from build123d import *

# Parameters (mm, degrees)
PAD_DEPTH = 3


with BuildPart() as part:
    # Sketch → Pad (new body, symmetric)
    with BuildSketch(Plane.XY):
        with BuildLine():
            Line((30, 12), (-30, 12))
            Line((-30, 12), (-30, 7))
            ThreePointArc((-30, 7), (-29.853553, 6.646447), (-29.5, 6.5))
            Line((-29.5, 6.5), (-28.829405, 6.5))
            ThreePointArc((-28.346442, 6.12941), (-28.525024, 6.396677), (-28.829405, 6.5))
            Line((-28.346442, 6.12941), (-25.908104, -2.97059))
            ThreePointArc((-26.391067, -3.6), (-25.99439, -3.404381), (-25.908104, -2.97059))
            Line((-27.753955, -3.6), (-26.391067, -3.6))
            Line((-29.62941, -3.097473), (-27.753955, -3.6))
            ThreePointArc((-30, -2.61451), (-29.896677, -2.918891), (-29.62941, -3.097473))
            Line((-30, -2.61451), (-30, -1))
            Line((-30, -1), (-31.6, -1))
            Line((-31.6, -1), (-31.6, -3))
            ThreePointArc((-31.6, -3), (-31.228036, -4.095771), (-30.265874, -4.738666))
            Line((-30.265874, -4.738666), (-25.68568, -5.965926))
            ThreePointArc((-25.68568, -5.965926), (-25.557387, -5.991445), (-25.426861, -6))
            Line((-25.426861, -6), (-19.034654, -6))
            ThreePointArc((-19.034654, -6), (-17.817131, -5.586707), (-17.102802, -4.517638))
            Line((-17.102802, -4.517638), (-16.5, -2.267949))
            Line((-16.5, -2.267949), (-16.5, -1.267949))
            Line((-16.5, -1.267949), (-17.5, -1))
            Line((-17.5, -1), (-17.5, 0))
            Line((-17.5, 0), (-16.5, 0))
            Line((-16.5, 0), (-16.5, 6.5))
            ThreePointArc((-15.5, 6.5), (-16, 7), (-16.5, 6.5))
            ThreePointArc((-15.5, 6.5), (-15.06066, 5.43934), (-14, 5))
            Line((-14, 5), (-11.154762, 5))
            ThreePointArc((-10.660644, 4.423529), (-10.775134, 4.825396), (-11.154762, 5))
            Line((-10.660644, 4.423529), (-11.5, -1))
            Line((-11.5, -1), (-11.5, -5))
            ThreePointArc((-11.5, -5), (-11.207107, -5.707107), (-10.5, -6))
            Line((-10.5, -6), (-8.5, -6))
            ThreePointArc((-8.5, -6), (-7.792893, -5.707107), (-7.5, -5))
            Line((-7.5, -5), (-7.5, -1))
            Line((-7.5, -1), (-6.964706, 2.458824))
            ThreePointArc((-4, 5), (-5.952374, 4.27777), (-6.964706, 2.458824))
            Line((-4, 5), (4, 5))
            ThreePointArc((6.964706, 2.458824), (5.952374, 4.27777), (4, 5))
            Line((6.964706, 2.458824), (7.5, -1))
            Line((7.5, -1), (7.5, -5))
            ThreePointArc((7.5, -5), (7.792893, -5.707107), (8.5, -6))
            Line((8.5, -6), (10.5, -6))
            ThreePointArc((10.5, -6), (11.207107, -5.707107), (11.5, -5))
            Line((11.5, -5), (11.5, -1))
            Line((11.5, -1), (10.815406, 3.423529))
            ThreePointArc((11.309524, 4), (10.929896, 3.825396), (10.815406, 3.423529))
            Line((11.309524, 4), (12, 4))
            ThreePointArc((12.5, 3.5), (12.353553, 3.853553), (12, 4))
            Line((12.5, 3.5), (12.5, 2))
            ThreePointArc((12.5, 2), (13.085786, 0.585786), (14.5, 0))
            Line((14.5, 0), (17.5, 0))
            Line((17.5, 0), (17.5, -1.2))
            Line((17.5, -1.2), (15.5, -1.7))
            Line((15.5, -1.7), (15.5, -2.5))
            Line((15.5, -2.5), (17.5, -3))
            Line((17.5, -3), (20.1, -3))
            ThreePointArc((20.1, -3), (20.701412, -2.907434), (21.247153, -2.638304))
            Line((21.247153, -2.638304), (27.272726, 1.580848))
            ThreePointArc((27.272726, 1.580848), (27.586161, 1.938251), (27.69915, 2.4))
            Line((27.69915, 2.4), (27.69915, 5))
            ThreePointArc((28.19915, 5.5), (27.845597, 5.353553), (27.69915, 5))
            Line((29, 5.5), (28.19915, 5.5))
            ThreePointArc((29, 5.5), (29.707107, 5.792893), (30, 6.5))
            Line((30, 6.5), (30, 12))
        make_face()
        with BuildLine():
            Line((-23.894296, -2.758819), (-26.409864, 6.62941))
            ThreePointArc((-26.409864, 6.62941), (-27.022236, 6.982963), (-27.37579, 6.37059))
            Line((-27.37579, 6.37059), (-24.527648, -4.258819))
            ThreePointArc((-24.527648, -4.258819), (-24.170484, -4.793353), (-23.561722, -5))
            Line((-23.561722, -5), (-19.061722, -5))
            ThreePointArc((-19.061722, -5), (-18.452961, -4.793353), (-18.095797, -4.258819))
            Line((-18.095797, -4.258819), (-17.5, -2.035276))
            Line((-17.5, -2.035276), (-18.5, -1.767327))
            Line((-18.5, -1.767327), (-18.5, 1))
            Line((-18.5, 1), (-17.5, 1))
            Line((-17.5, 1), (-17.5, 6.5))
            ThreePointArc((-17.5, 6.5), (-17.646447, 6.853553), (-18, 7))
            Line((-18, 7), (-19.5, 7))
            ThreePointArc((-19.5, 7), (-19.853553, 6.853553), (-20, 6.5))
            Line((-20, 6.5), (-20, -2.5))
            ThreePointArc((-21, -3.5), (-20.292893, -3.207107), (-20, -2.5))
            Line((-21, -3.5), (-22.92837, -3.5))
            ThreePointArc((-23.894296, -2.758819), (-23.537131, -3.293353), (-22.92837, -3.5))
        make_face(mode=Mode.SUBTRACT)
        with BuildLine():
            Line((25.818763, 4), (13.7, 4))
            Line((13.7, 4), (13.7, 2))
            ThreePointArc((13.7, 2), (13.934315, 1.434315), (14.5, 1.2))
            Line((14.5, 1.2), (18.7, 1.2))
            Line((18.7, 1.2), (18.7, -1.8))
            Line((18.7, -1.8), (20.1, -1.8))
            ThreePointArc((20.1, -1.8), (20.400706, -1.753717), (20.673576, -1.619152))
            Line((20.673576, -1.619152), (25.477624, 1.744678))
            ThreePointArc((25.477624, 1.744678), (25.728372, 2.030601), (25.818763, 2.4))
            Line((25.818763, 2.4), (25.818763, 4))
        make_face(mode=Mode.SUBTRACT)
    extrude(amount=PAD_DEPTH, both=True)


solid = part.part
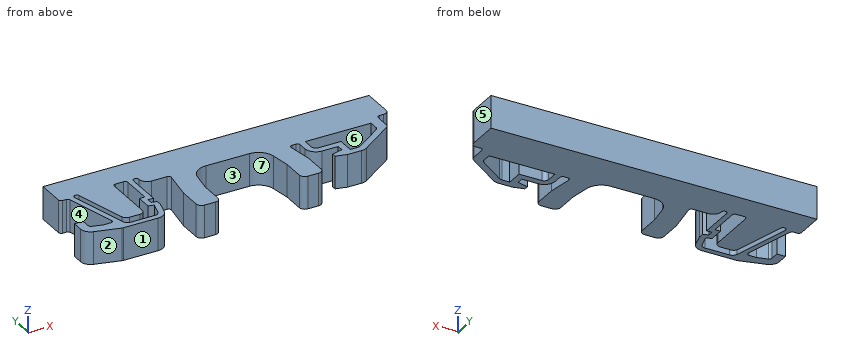
The listing builds one solid part. Answer for the finished solid, in the listing's coordinates (mm). Face numbers are marked on the shaded views. A direction names the side the tool comes from. Round coordinates to 2 decimals unless told otherwise and drop trailing zeros. Write each loop counter-clockwise with the first axis right and the second up, starting at its lowest first coordinate (ties: lowest second). Pieces come first, ordered by that corner, then holes. Notation, with made-up numbers: (-39.5, 6.25) - (-17.5, 6.25) arc R27 cw to (-17.5, 45.25) - close; hole circle Ø5 at (-40, 89.25). An arc over 180 degrees is marked (long way). Use one line per item in the form item = value. Start each with the question number.
Item 1: A tool of negligible diameter and unlimited length cuts with its end or side. For the marked faces 5, 6 and 7, from which of +Z, -Z, +X, -X, +Y, -Y can it reach the whole face along a straight path? Write none if from no direction.
Item 2: Find the intervals of material crossed by line 1 (X direction, y = 4.5, z = -1.65); line 2 (Y direction, x = 18, z = 1.6); line 3 (Y direction, x = -12, z = 1.9), in increasing order. Write a range as [from, to].
Item 3: Flat-ended cylindrical pins translate along their axes: pin 1 Ø1.3 at (y, z) = (3, 0.5) entering from +X; pin 2 Ø3 at (x, z) = (18.5, -1) entering from -Y; pin 3 Ø0.5 at (y, z) = (-0.5, -1.5) entering from +X. Find the tip coordinate at first contact, or state that the pin passes through.
Item 4: Determine the mould class of the marked faces 1, 2, 3 and 4 for opening direction X: +X half, -X half, draft (parallel to the pull), parting line (faces both ways), or undercut.
Item 5: A cutting plane is placed at A-A (z = 0.45). Give the number of separate pieces and of enclosed holes in the cut face, plus the area to 3 significant figures.
Item 6: A cutting plane is placed at B-B (y = 10). Write down the section's boundary in (x, z), plus the area to 3 significant figures.
The answers:
q1.face_5 = +Z, -Z, +X, +Y, -Y
q1.face_6 = +Z, -Z
q1.face_7 = +Z, -Z, -Y
q2.line_1 = [-27.91, -26.87], [-25.84, -20], [-17.5, -16.5], [-10.65, -5.66], [5.66, 27.7]
q2.line_2 = [-3, 1.2], [4, 12]
q2.line_3 = [5, 12]
q3.pin_1 = 27.7
q3.pin_2 = -3
q3.pin_3 = 24.66
q4.face_1 = draft
q4.face_2 = -X half
q4.face_3 = undercut
q4.face_4 = undercut
q5.separate_pieces = 1
q5.enclosed_holes = 2
q5.area = 630 mm^2
q6.outline = (-30, -3) - (30, -3) - (30, 3) - (-30, 3) - close
q6.area = 360 mm^2
